from build123d import *

# Parameters (mm, degrees)
BOSS_EXTRUDE1_DEPTH     = 30.48
CUT_EXTRUDE1_DEPTH      = 42.659097446
CUT_EXTRUDE1_DEPTH_BACK = 42.659097446
SKETCH3_W               = 25.4
SKETCH3_H               = 12.7


with BuildPart() as part:
    # Sketch2 → Boss-Extrude1 (new body)
    with BuildSketch(Plane.XY):
        with BuildLine():
            Line((-12.7, 0), (-12.7, -12.7))
            Line((-12.7, -12.7), (12.7, -12.7))
            Line((12.7, -12.7), (12.7, 0))
            ThreePointArc((12.7, 0), (0, 12.7), (-12.7, 0))
        make_face()
    extrude(amount=BOSS_EXTRUDE1_DEPTH)

    # Sketch3 → Cut-Extrude1 (cut, two sides: drawn at the far end of the back side and taken through both)
    with BuildSketch(Plane(origin=(12.7, 0, 0), x_dir=(0, 0, -1), z_dir=(1, 0, 0)).offset(-CUT_EXTRUDE1_DEPTH_BACK)):
        with Locations((-15.24, 6.35)):
            Rectangle(SKETCH3_W, SKETCH3_H)
    extrude(amount=CUT_EXTRUDE1_DEPTH + CUT_EXTRUDE1_DEPTH_BACK, mode=Mode.SUBTRACT)


solid = part.part
Here's how the part is built. I have some questions about the finished solid (model axes, mm). A direction names the side the tool comes from. Coordinates: 2 decimals unless noted, no trailing zeros. Order: outer loops, then holes, each group sorted by start corner. A loop starts at its lowest first (then second) coordinate and runs counter-clockwise, first axis right, second up.
Item 1: If we section it at B-B on x = 0: List the corners of the cut face in (y, z) for me, plus the area to 3 significant figures.
Result sheet:
outline: (-12.7, 0) - (12.7, 0) - (12.7, 2.54) - (0, 2.54) - (0, 27.94) - (12.7, 27.94) - (12.7, 30.48) - (-12.7, 30.48) - close
area: 452 mm2
Item 2: If we section it at A-A on y = 4.25: List the corners of the cut face in (x, z) for me.
Result sheet:
outline: (-11.97, 0) - (11.97, 0) - (11.97, 2.54) - (-11.97, 2.54) - close; (-11.97, 27.94) - (11.97, 27.94) - (11.97, 30.48) - (-11.97, 30.48) - close
Item 3: If we mould it in two halves opening along Z, with no side actions, what happens to faces 1 (the face through (0, 0, 15)), 2 (the face through (0, 0, 0)), 3 (the face through (0.279, 12.697, 29.192))? For each: +Z half, -Z half, draft (parallel to the pull), parting line (faces both ways), or undercut.
Result sheet:
face 1: undercut
face 2: -Z half
face 3: draft
Item 4: If we section it at C-C on z = 11.5: List the corners of the cut face in (x, y) for me.
Result sheet:
outline: (-12.7, -12.7) - (12.7, -12.7) - (12.7, 0) - (-12.7, 0) - close
Item 5: For P1, Ø1.5, axis at x = 2, z = 26.5, coming from the +Y side; P2, Ø10, axis at x = 8.5, y = -5, coming from the -Z side, each with a flat end and sliding along its axis, tell me the tip position at first contact or that it passes through.
Result sheet:
P1: stops at y = 0
P2: stops at z = 0
Item 6: I need wall thicknesses on line 1 (Z direction, x = 3.75, y = 3.5); line 2 (Y direction, x = 6, z = 23); line 3 (Y direction, x = -5.5, z = 28). Which ranges of each line are inside material? Lowest first, please.
Result sheet:
line 1: z = 0 to 2.54, 27.94 to 30.48
line 2: y = -12.7 to 0
line 3: y = -12.7 to 11.45
Item 7: For faces 4 (the face through (12.7, -6, 15)), 5 (the face through (0, 5, 27.94)), which set-ups out of +Z, -Z, +X, -X, +Y, -Y let a thin tool reach every point of the face, with its end or its side?
Result sheet:
face 4: +Z, -Z, +X, +Y, -Y
face 5: +X, -X, +Y
Item 8: If we section it at D-D on y = 0.5: List the corners of the cut face in (x, z) for me.
Result sheet:
outline: (-12.69, 0) - (12.69, 0) - (12.69, 2.54) - (-12.69, 2.54) - close; (-12.69, 27.94) - (12.69, 27.94) - (12.69, 30.48) - (-12.69, 30.48) - close
